from build123d import *

# Parameters (mm, degrees)
SKETCH1_W           = 100
SKETCH1_H           = 79
SKETCH1_R           = 1.375
BOSS_EXTRUDE1_DEPTH = 1.57
SKETCH2_W           = 73
SKETCH2_H           = 50
BOSS_EXTRUDE2_DEPTH = 26.706


with BuildPart() as part:
    # Sketch1 → Boss-Extrude1 (new body)
    with BuildSketch(Plane(origin=(0, 0, 0), x_dir=(1, 0, 0), z_dir=(0, 1, 0))):
        Rectangle(SKETCH1_W, SKETCH1_H)
        with Locations((-46, 35.5)):
            Circle(SKETCH1_R, mode=Mode.SUBTRACT)
        with Locations((40, 35.5)):
            Circle(SKETCH1_R, mode=Mode.SUBTRACT)
        with Locations((-46, -22.5)):
            Circle(SKETCH1_R, mode=Mode.SUBTRACT)
        with Locations((40, -22.5)):
            Circle(SKETCH1_R, mode=Mode.SUBTRACT)
    extrude(amount=BOSS_EXTRUDE1_DEPTH)

    # Sketch2 → Boss-Extrude2 (add)
    with BuildSketch(Plane(origin=(0, 1.57, 0), x_dir=(1, 0, 0), z_dir=(0, 1, 0))):
        with Locations((-2, 14)):
            Rectangle(SKETCH2_W, SKETCH2_H)
    extrude(amount=BOSS_EXTRUDE2_DEPTH)


solid = part.part
Input: part model. Units: mm. Frame: model coordinates. A direction names the side the tool comes from. Coordinates: 2 decimals unless noted, no trailing zeros. Loops run counter-clockwise (first coordinate to the right, second up) from the corner with the lowest first, then second, coordinate; pieces in that order, holes last. Notation, with made-up numbers: (-1, 21) - (51, 21) arc R13 ccw to (51, 26) - close; hole circle Ø10 at (-6.75, 44.5). An arc over 180 degrees is marked (long way). Answer in a Markdown table with one row per item. Add a question column.
Item 1: Contact query for flat-ended pins moving along their axis: P1, Ø12, axis at y = 20, z = -2, coming from the -X side; P2, Ø3, axis at x = -46, z = 22.5, coming from the +Y side; P3, Ø8, axis at y = 24, z = -3.5, coming from the +X side. Output: stop coordinate, or through.
Item 2: Section query D-D on z = 2. Return the cut outline in (x, y), then the cut area to 3 significant figures.
Item 3: Section query C-C on x = 28. Return the cut outline in (y, z).
Item 4: Section query B-B on x = 40. Return the cut outline in (y, z) (3 decimals), then the cut area to 3 significant figures.
Item 5: Section query A-A on z = -35.5. Return the cut outline in (x, y) (3 decimals), then the cut area to 3 significant figures.
Item 6: Line query: line 1 along X through (y, z) = (0.85, -35.5) (3 decimals); line 2 along Z through (x, y) = (40, 1.2) (3 decimals); line 3 along Y through (x, z) = (21, 14). Output: solid intervals per line, ascending. Write a range as [from, to].
Item 7: Mould query, pull axis Z, two halves, no side actions, for faces 1 (the cylindrical face through (38.987, 0.774, -36.429)), 2 (the flat face through (34.5, 15, -14)), 3 (the flat face through (-3, 15, 11)), 4 (the cylindrical face through (38.626, 0.774, 22.44)). Classes: released by +Z, released by -Z, zero draft, split by the parting line, or undercut.
Item 8: Access query for faces 5 (the flat face through (-3, 15, -39)), 6 (the flat face through (-38.5, 15, -14)), 7 (the cylindrical face through (-47.374, 0.774, 22.44)). Directions: +Z, -Z, +X, -X, +Y, -Y. A direction counts if a zero-diameter tool reaches every point of the face in a straight line with its end or side. Return the directions, or none.
Recorded:
| question | item | result |
|---|---|---|
| 1 | P1 | x = -38.5 |
| 1 | P2 | y = 1.57 |
| 1 | P3 | x = 34.5 |
| 2 | outline | (-50, 0) - (50, 0) - (50, 1.57) - (34.5, 1.57) - (34.5, 28.28) - (-38.5, 28.28) - (-38.5, 1.57) - (-50, 1.57) - close |
| 2 | area | 2,110 mm^2 |
| 3 | outline | (0, -39.5) - (1.57, -39.5) - (1.57, -39) - (28.28, -39) - (28.28, 11) - (1.57, 11) - (1.57, 39.5) - (0, 39.5) - close |
| 4 | outline | (0, -39.5) - (1.57, -39.5) - (1.57, -36.875) - (0, -36.875) - close; (0, -34.125) - (1.57, -34.125) - (1.57, 21.125) - (0, 21.125) - close; (0, 23.875) - (1.57, 23.875) - (1.57, 39.5) - (0, 39.5) - close |
| 4 | area | 115 mm^2 |
| 5 | outline | (-50, 0) - (-47.375, 0) - (-47.375, 1.57) - (-50, 1.57) - close; (-44.625, 0) - (38.625, 0) - (38.625, 1.57) - (34.5, 1.57) - (34.5, 28.276) - (-38.5, 28.276) - (-38.5, 1.57) - (-44.625, 1.57) - close; (41.375, 0) - (50, 0) - (50, 1.57) - (41.375, 1.57) - close |
| 5 | area | 2,100 mm^2 |
| 6 | line 1 | [-50, -47.375], [-44.625, 38.625], [41.375, 50] |
| 6 | line 2 | [-39.5, -36.875], [-34.125, 21.125], [23.875, 39.5] |
| 6 | line 3 | [0, 1.57] |
| 7 | face 1 | undercut |
| 7 | face 2 | zero draft |
| 7 | face 3 | released by +Z |
| 7 | face 4 | undercut |
| 8 | face 5 | -Z, +X, -X, +Y |
| 8 | face 6 | +Z, -Z, -X, +Y |
| 8 | face 7 | +Y, -Y |
